```python
from build123d import *

# Parameters (mm, degrees)
IZIM1_W                     = 100
IZIM1_H                     = 50
Y_KSEKLIK_EKSTR_ZYON1_DEPTH = 80
IZIM2_W                     = 40
IZIM2_H                     = 40
Y_KSEKLIK_EKSTR_ZYON6_DEPTH = 150
KES_EKSTR_ZYON4_DEPTH       = 50
IZIM12_R                    = 5
Y_KSEKLIK_EKSTR_ZYON9_DEPTH = 5
IZIM13_R                    = 23
KES_EKSTR_ZYON9_DEPTH       = 78
IZIM14_R                    = 2
KES_EKSTR_ZYON10_DEPTH      = 78
IZIM15_W                    = 16.621675202
IZIM15_H                    = 40
KES_EKSTR_ZYON15_DEPTH      = 20


with BuildPart() as part:
    # Çizim1 → Yükseklik-Ekstrüzyon1 (new body)
    with BuildSketch(Plane.XY):
        with Locations((-50, -0.013722327)):
            Rectangle(IZIM1_W, IZIM1_H)
    extrude(amount=Y_KSEKLIK_EKSTR_ZYON1_DEPTH)

    # Çizim2 → Yükseklik-Ekstrüzyon6 (add)
    with BuildSketch(Plane(origin=(0, 0, 0), x_dir=(0, 1, 0), z_dir=(0.7071067811865561, 0, 0.7071067811865389))):
        with Locations((-1.342558947, 32.385430267)):
            Rectangle(IZIM2_W, IZIM2_H)
    extrude(amount=Y_KSEKLIK_EKSTR_ZYON6_DEPTH)

    # Çizim11 → Kes-Ekstrüzyon4 (cut)
    with BuildSketch(Plane(origin=(0, 0, 114.823838907), x_dir=(0, 1, 0), z_dir=(0, 0, 1))):
        Polygon((18.657441053, -97.308195449), (-21.342558947, -97.308195449), (-41.210000873, -31.823007329), (29.36267087, -31.823007329), align=None)
    extrude(amount=KES_EKSTR_ZYON4_DEPTH, mode=Mode.SUBTRACT)

    # Çizim12 → Yükseklik-Ekstrüzyon9 (add)
    with BuildSketch(Plane.XY.offset(114.823838907)):
        with Locations(Location((69.745895445, -1.722983567, 0), (0, 0, 180))):
            Circle(IZIM12_R)
    extrude(amount=Y_KSEKLIK_EKSTR_ZYON9_DEPTH)

    # Çizim13 → Kes-Ekstrüzyon9 (cut)
    with BuildSketch(Plane.XY.offset(80)):
        with Locations((-75, -0.013722327)):
            Circle(IZIM13_R)
    extrude(amount=-KES_EKSTR_ZYON9_DEPTH, mode=Mode.SUBTRACT)

    # Çizim14 → Kes-Ekstrüzyon10 (cut)
    with BuildSketch(Plane(origin=(0, 0, 0), x_dir=(-1, 0, 0), z_dir=(0, 0, -1))):
        with Locations((75, -0.013722327)):
            Circle(IZIM14_R)
    extrude(amount=-KES_EKSTR_ZYON10_DEPTH, mode=Mode.SUBTRACT)

    # Çizim15 → Kes-Ekstrüzyon15 (cut)
    with BuildSketch(Plane.XY.offset(114.823838907)):
        with Locations((88.997357848, -1.342558947)):
            Rectangle(IZIM15_W, IZIM15_H)
    extrude(amount=-KES_EKSTR_ZYON15_DEPTH, mode=Mode.SUBTRACT)


solid = part.part
```
Part model, mm, in its own coordinate system. A direction names the side the tool comes from. Round coordinates to 2 decimals unless told otherwise and drop trailing zeros. Loops run counter-clockwise (first coordinate to the right, second up) from the corner with the lowest first, then second, coordinate; pieces in that order, holes last. Notation, with made-up numbers: (61, -11.75) -> (102, -11.75) arc R24 ccw to (102, 6.25) -> close; hole circle Ø11 at (17, 36.5). An arc over 180 degrees is marked (long way). Use one line per item in the form item = value. Start each with the question number.
Item 1: Band-saw the part on A-A (x = -75). List the corners of the cut face in (y, z).
Item 2: Two-plate mould, pull along X, no slides. Class faces 1 (the flat face through (60, -1, 114.824)), 2 (the flat face through (80.687, -2, 107)), 3 (the flat face through (0, 0, 13)), 4 (the flat face through (-100, 0, 39)): released by +X, released by -X, zero draft, split by the parting line, or undercut.
Item 3: Band-saw the part on C-C (x = -25). List the corners of the cut face in (y, z), plus the area to 3 significant figures.
Item 4: Drop flat-ended pins along their axis: pin 1 Ø5 at (x, y) = (-31, -2) entering from -Z; pin 2 Ø24 at (x, z) = (21, 50) entering from +Y; pin 3 Ø20 at (x, y) = (53.5, -5) entering from +Z; pin 4 Ø14 at (x, y) = (-65.5, -1.5) entering from +Z. Give the stop position or say it passes through.
Item 5: Drill centre lines: line 1 along Y through (x, z) = (-75, 31); line 2 along X through (y, z) = (14.5, 77); line 3 along Z through (x, y) = (-8, -15.5). Where is each one in solid material? Low to high.
Item 6: Tool access for faces 5 (the flat face through (-51, 0, 0)), 6 (the flat face through (30, 18.657, 75)), 7 (the flat face through (30, -21.343, 75)), 8 (the flat face through (-75, -5, 2)), 9 (the flat face through (-40, 0, 80)): list every direction of +Z, -Z, +X, -X, +Y, -Y with a clear straight run to the whole face (end or side of a thin tool).
Item 7: Band-saw the part on D-D (z = 12.5). List the corners of the cut face in (x, y), plus the area to 3 significant figures.
Item 8: Band-saw the part on B-B (z = 30). List the corners of the cut face in (x, y), plus the area to 3 significant figures.
Data:
q1.outline = (-25.01, 0) -> (-2.01, 0) -> (-2.01, 2) -> (-23.01, 2) -> (-23.01, 80) -> (-25.01, 80) -> close; (1.99, 0) -> (24.99, 0) -> (24.99, 80) -> (22.99, 80) -> (22.99, 2) -> (1.99, 2) -> close
q2.face_1 = zero draft
q2.face_2 = released by +X
q2.face_3 = undercut
q2.face_4 = released by -X
q3.outline = (-25.01, 0) -> (24.99, 0) -> (24.99, 80) -> (-25.01, 80) -> close
q3.area = 4,000 mm^2
q4.pin_1 = 0
q4.pin_2 = 18.66
q4.pin_3 = 114.82
q4.pin_4 = 2
q5.line_1 = -25.01 to -23.01, 22.99 to 24.99
q5.line_2 = -100 to -92.84, -57.16 to 0, 2.92 to 59.48
q5.line_3 = 0 to 80
q6.face_5 = -Z, +X, -X, +Y, -Y
q6.face_6 = +Z, -Z, +X, +Y
q6.face_7 = +Z, -Z, +X, -Y
q6.face_8 = +Z
q6.face_9 = +Z, -X, +Y, -Y
q7.outline = (-100, -25.01) -> (0, -25.01) -> (0, 24.99) -> (-100, 24.99) -> close; hole circle Ø46 at (-75, -0.01)
q7.area = 3,340 mm^2
q8.outline = (-100, -25.01) -> (0, -25.01) -> (0, -21.34) -> (12.48, -21.34) -> (12.48, 18.66) -> (0, 18.66) -> (0, 24.99) -> (-100, 24.99) -> close; hole circle Ø46 at (-75, -0.01)
q8.area = 3,840 mm^2
